Geometry: final body of the model. Coordinates: model frame, mm. Coordinates: 2 decimals unless noted, no trailing zeros. Write each loop counter-clockwise with the first axis right and the second up, starting at its lowest first coordinate (ties: lowest second). Pieces come first, ordered by that corner, then holes. Notation, with made-up numbers: M 75,75.5 L 119,75.5 A10 cw 119,88.5 Z; hole C -28.75,-5.5 d8. An arc over 180 degrees is marked long. Write item = value, one per line. Start each with the question number.
Item 1: Ray query, L1, parallel to Z at x = 0, y = 2.4; L2, parallel to Z at x = 1, y = 0.2; L3, parallel to X at y = 2.9, z = -0.25. Return the intervals inside material, ascending. Write a range as [from, to].
Item 2: Pull-direction query (X, two-part tool) for faces 1 (the cylindrical face through (-3.352, 1.863, -2.524)), 2 (the cylindrical face through (-1.873, 1.849, -0.082)), 3 (the cylindrical face through (-0.14, 1.86, 6.25)), 4 (the flat face through (-0.1, 0, 2.3)); classes: +X half, -X half, draft (parallel to the pull), parting line (faces both ways), or undercut.
Item 3: Section B-B on y = 1.8. Output: boundary loops of the cut face in (x, z) (3 decimals).
Item 4: Section A-A on x = 0. Output: boundary loops of the cut face in (y, z), plus the area to 3 significant figures.
Item 5: Section C-C on y = 2.9. Output: boundary loops of the cut face in (x, z) (3 decimals).
Item 6: First-contact query: pin 1 Ø2 at (x, z) = (-4.5, 4.5) entering from +Y. Flat tip, straight axial feed; report the tip coordinate or a pass-through.
from build123d import *

# Parameters (mm, degrees)
SKETCH1_R           = 1.875
SKETCH1_R_2         = 0.935
BOSS_EXTRUDE1_DEPTH = 3.75
FILLET1_R           = 1
FILLET2_R           = 1


with BuildPart() as part:
    # Sketch1 → Boss-Extrude1 (new body)
    with BuildSketch(Plane(origin=(0, 0, 0), x_dir=(1, 0, 0), z_dir=(0, 1, 0))):
        with BuildLine():
            ThreePointArc((-6.25, 0), (0, -6.250030085), (6.25, 0))
            ThreePointArc((6.25, 0), (3.383257686, 2.480432696), (1.88, 5.960515192))
            ThreePointArc((1.88, 5.960515192), (0, 6.249969915), (-1.88, 5.960515192))
            ThreePointArc((-1.88, 5.960515192), (-3.383257686, 2.480432696), (-6.25, 0))
        make_face()
        with Locations((0, -3.0085e-05)):
            Circle(SKETCH1_R, mode=Mode.SUBTRACT)
        with Locations((0, 3.749969915)):
            Circle(SKETCH1_R_2, mode=Mode.SUBTRACT)
    extrude(amount=BOSS_EXTRUDE1_DEPTH)

    # Fillet1
    fillet1_edges = [part.edges().sort_by_distance(p)[0] for p in [
        (3.383257686, 3.75, -2.480432696),
        (0, 3.75, -6.249969915),
        (-3.383257686, 3.75, -2.480432696),
        (0, 3.75, 6.250030085),
    ]]
    fillet(fillet1_edges, radius=FILLET1_R)

    # Fillet2
    fillet2_edges = [part.edges().sort_by_distance(p)[0] for p in [
        (0, 0, -6.249969915),
        (3.383257686, 0, -2.480432696),
        (0, 0, 6.250030085),
        (-3.383257686, 0, -2.480432696),
    ]]
    fillet(fillet2_edges, radius=FILLET2_R)


solid = part.part
Responses:
q1.L1 = [-6.25, -4.68], [-2.81, -1.87], [1.88, 6.25]
q1.L2 = [-5.76, -1.59], [1.59, 5.76]
q1.L3 = [-5.79, -1.86], [1.86, 5.79]
q2.face_1 = -X half
q2.face_2 = undercut
q2.face_3 = parting line
q2.face_4 = draft
q3.outline = M -6.25,0 A8.5 cw -1.88,-5.961 A6.25 ccw 1.88,-5.961 A8.5 cw 6.25,0 A6.25 ccw Z; hole C 0,0 d3.75; hole C 0,-3.75 d1.87
q4.outline = M 0,-5.25 A1 ccw 1,-6.25 L 2.75,-6.25 A1 ccw 3.75,-5.25 L 3.75,-4.68 L 0,-4.68 Z; M 0,-2.81 L 3.75,-2.81 L 3.75,-1.87 L 0,-1.87 Z; M 0,1.88 L 3.75,1.88 L 3.75,5.25 A1 ccw 2.75,6.25 L 1,6.25 A1 ccw 0,5.25 Z
q4.area = 24.9 mm²
q5.outline = M -6.239,0.007 A8.511 cw -1.87,-5.952 A6.239 ccw 1.87,-5.952 A8.511 cw 6.239,0.007 A6.239 ccw Z; hole C 0,0 d3.75; hole C 0,-3.75 d1.87
q6.pin_1 = 3.74
